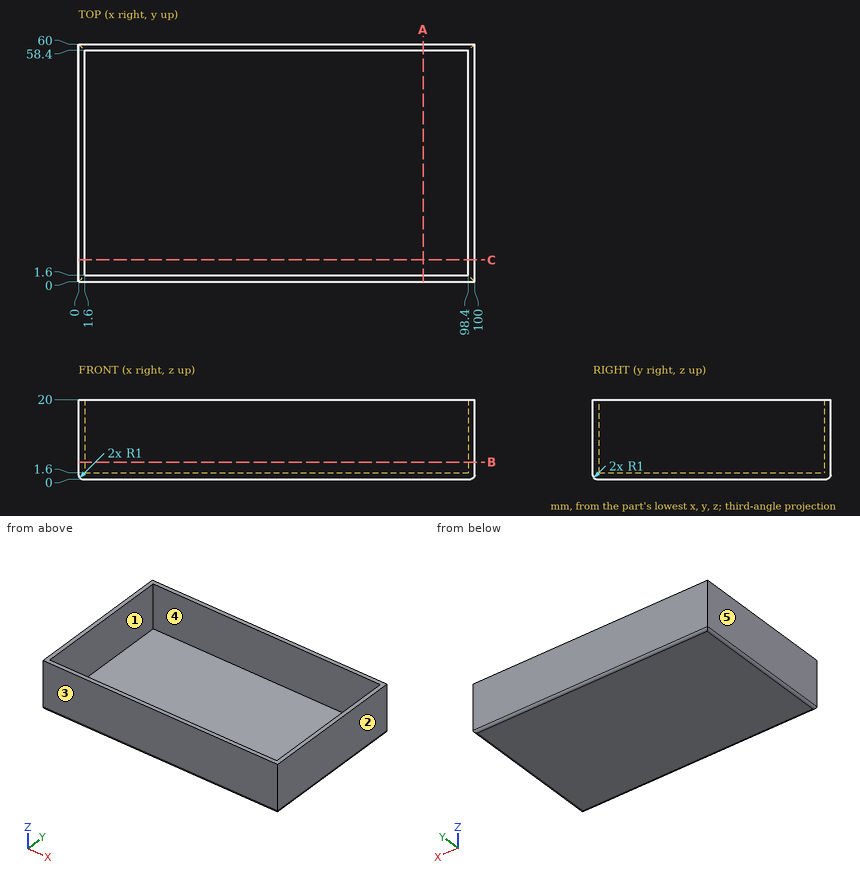
Here's the drawing with two shaded views (mm, measured from the low corner). I have some questions. A direction names the side the tool comes from. Round coordinates to 2 decimals unless told otherwise and drop trailing zeros. Write each loop counter-clockwise with the first axis right and the second up, starting at its lowest first coordinate (ties: lowest second). Pieces come first, ordered by that corner, then holes. Notation, with made-up numbers: M -14.75,15.5 L 6.25,15.5 A34 cw 6.25,54.5 Z; hole C 70,15 d7. An arc over 180 degrees is marked long. Answer in a Markdown table with one row per item. Add a question column.
Q1. Imagine slicing it at B-B (z = 4.25). Please give me the cut outline in (x, y).
Q2. If I drill on line 1 (X direction, y = 4, z = 17.25); line 2 (Y direction, x = 19.5, z = 3.75); line 3 (Z direction, x = 54, y = 24.5), over which ranges is the centre line in solid material (lowest first)? Write a range as from..to.
Q3. On a 3-axis mill with a long thin cutter (end or side, diameter ignored), from which of +Z, -Z, +X, -X, +Y, -Y can I reach the whole of each face in a straight line? I mean the marked faces 4 and 5. Say none if no direction works.
Q4. Imagine slicing it at C-C (y = 5.5). Please give me the cut outline in (x, z).
Q5. If we mould it in two halves opening along X, with no side actions, what happens to the marked faces 1, 2 and 3? For each: +X half, -X half, draft (parallel to the pull), parting line (faces both ways), or undercut.
Q6. Will this pin go through, and if not, where does the flat tip stop? pin 1 Ø3 at (x, y) = (29, 15.5) entering from +Z.
Q7. Imagine slicing it at A-A (x = 87). Please give me the cut outline in (y, z), then the cut area to 3 significant figures.
Values:
| question | item | result |
|---|---|---|
| 1 | outline | M 0,0 L 100,0 L 100,60 L 0,60 Z; hole M 1.6,1.6 L 98.4,1.6 L 98.4,58.4 L 1.6,58.4 Z |
| 2 | line 1 | 0..1.6, 98.4..100 |
| 2 | line 2 | 0..1.6, 58.4..60 |
| 2 | line 3 | 0..1.6 |
| 3 | face 4 | +Z |
| 3 | face 5 | +Z, -Z, -X, +Y, -Y |
| 4 | outline | M 0,1 A1 ccw 1,0 L 99,0 A1 ccw 100,1 L 100,20 L 98.4,20 L 98.4,1.6 L 1.6,1.6 L 1.6,20 L 0,20 Z |
| 5 | face 1 | undercut |
| 5 | face 2 | +X half |
| 5 | face 3 | draft |
| 6 | pin 1 | z = 1.6 |
| 7 | outline | M 0,1 A1 ccw 1,0 L 59,0 A1 ccw 60,1 L 60,20 L 58.4,20 L 58.4,1.6 L 1.6,1.6 L 1.6,20 L 0,20 Z |
| 7 | area | 154 mm^2 |
